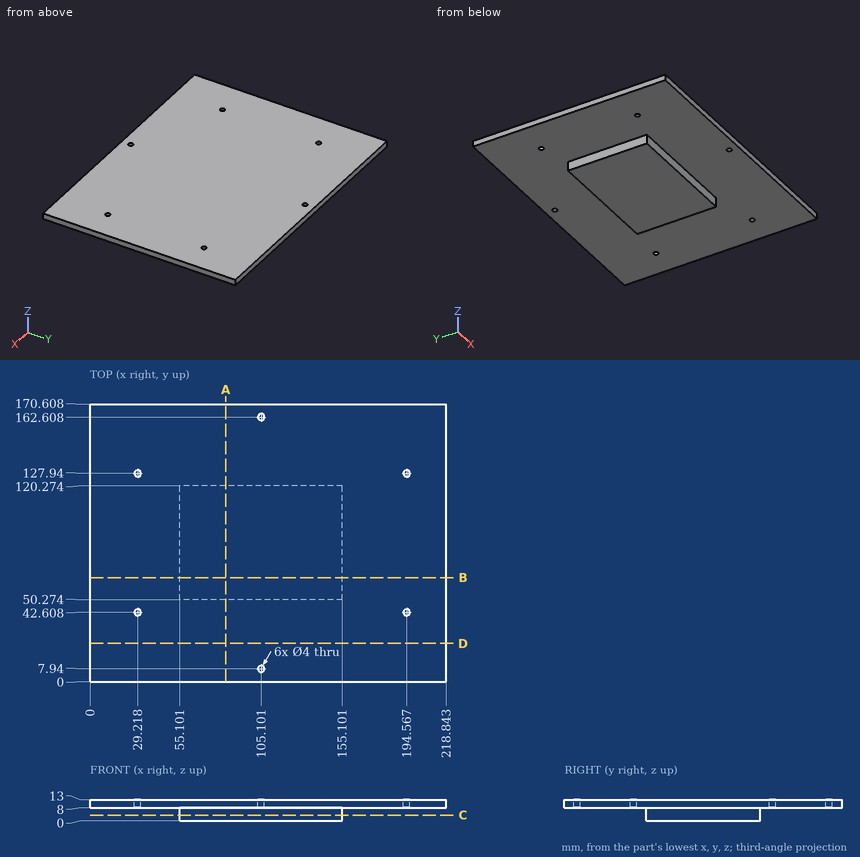
The figure shows three views and two pictorial views of one solid part (mm, origin at its lowest corner). Answer the questions. Round coordinates to 2 decimals unless told otherwise and drop trailing zeros. Loops run counter-clockwise (first coordinate to the right, second up) from the corner with the lowest first, then second, coordinate; pieces in that order, holes last. Notation, with made-up numbers: (29, -14.5) - (43, -14.5) arc R10 cw to (43, -1.5) - close; hole circle Ø8 at (4, 21.25). An arc over 180 degrees is marked (long way). Use one line per item in the form item = value. Start each with the question number.
(1) Find section D-D on y = 23.5. Determine the outline of the cut face in (x, z).
(2) Consider line 1 (X direction, y = 127.94, z = 11.3); line 2 (X direction, y = 7.94, z = 10.7); line 3 (Z direction, x = 22.5, y = 51). Determine where each line is inside the solid, lowest interval first.
(3) Find section B-B on y = 64. Determine the outline of the cut face in (x, z).
(4) Find section C-C on z = 3.5. Determine the outline of the cut face in (x, y).
(5) Find section A-A on x = 83.5. Determine the outline of the cut face in (y, z), and give its area (3 significant figures).
(6) Flat-ended cylindrical pins translate along their axes: P1, Ø2.5, axis at y = 73, z = 3, coming from the +X side; P2, Ø6.5, axis at x = 105.1, y = 7.94, coming from the -Z side; P3, Ø3.5, axis at x = 29.22, y = 42.61, coming from the +Z side; P4, Ø2.5, axis at x = 108, z = 5.5, coming from the +Y side. Find the tip coordinate at first contact, or state that the pin passes through.
Answer list:
q1.outline = (0, 8) - (218.84, 8) - (218.84, 13) - (0, 13) - close
q2.line_1 = 0 to 27.22, 31.22 to 192.57, 196.57 to 218.84
q2.line_2 = 0 to 103.1, 107.1 to 218.84
q2.line_3 = 8 to 13
q3.outline = (0, 8) - (55.1, 8) - (55.1, 0) - (155.1, 0) - (155.1, 8) - (218.84, 8) - (218.84, 13) - (0, 13) - close
q4.outline = (55.1, 50.27) - (155.1, 50.27) - (155.1, 120.27) - (55.1, 120.27) - close
q5.outline = (0, 8) - (50.27, 8) - (50.27, 0) - (120.27, 0) - (120.27, 8) - (170.61, 8) - (170.61, 13) - (0, 13) - close
q5.area = 1,410 mm^2
q6.P1 = 155.1
q6.P2 = 8
q6.P3 = through
q6.P4 = 120.27
